Here's how the part is built. I have some questions about the finished solid (model axes, mm). A direction names the side the tool comes from. Coordinates: 2 decimals unless noted, no trailing zeros. Order: outer loops, then holes, each group sorted by start corner. A loop starts at its lowest first (then second) coordinate and runs counter-clockwise, first axis right, second up. Notation, with made-up numbers: (8.25, -39) - (47.25, -39) arc R26 cw to (47.25, -6) - close; hole circle Ø6 at (15.25, 89). An arc over 180 degrees is marked (long way). Answer as CSV lines item,"result". Start each with the question number.
Item 1: Imagine slicing it at C-C on z = -2. List the corners of the cut face in (x, y) for me.
Item 2: Imagine slicing it at A-A on x = 11.5. List the corners of the cut face in (y, z) for me.
Item 3: Imagine slicing it at B-B on y = 2.4. List the corners of the cut face in (x, z) for me.
Item 4: I need wall thicknesses on line 1 (Z direction, x = 11, y = 0.9); line 2 (Z direction, x = 14.5, y = 1.05); line 3 (X direction, y = 2.45, z = -16.5). Which ranges of each line are inside material? Lowest first, please.
Item 5: We'd pull the mould along X, two halves only. Please class faces 5 (the face through (10.762, 1, -62)), 6 (the face through (-18.42, 1.521, -50.347)), 7 (the face through (-19.238, 1, -70)), 8 (the face through (14.566, 1.521, -50.326)): pulls with the +X half, pulls with the -X half, needs draft (parallel to the pull), parting line crosses it, or undercut.
Item 6: I'm going to push flat-ended pins straight in: pin 1 (1.5 mm diameter, centred on y = 1.5, z = -69.5, fed in from +X); pin 2 (1.5 mm diameter, centred on y = 1, z = -9, fed in from -X); pin 3 (3.5 mm diameter, centred on x = -2.74, z = 0.94, fed in from -Y); pin 4 (1.5 mm diameter, centred on x = 12, y = 2, fed in from +Z). Where does each tip first touch, or does it pass through?
Item 7: On a 3-axis mill with a long thin cutter (end or side, diameter ignored), from which of +Z, -Z, +X, -X, +Y, -Y can I reach the whole of each face in a straight line? I mean faces 1 (the face through (14, 1, -56.064)), 2 (the face through (13.762, 1, -70)), 3 (the face through (-19, 1, -44.064)), 4 (the face through (-19, 1, -56.064)). Say none if no direction works.
Autodesk Inventor part; units mm, degrees
ref_plane "YZ Plane" through (0, 0, 0) normal (1, 0, 0) x (0, 1, 0)
ref_plane "XZ Plane" through (0, 0, 0) normal (0, 1, 0) x (-1, 0, 0)
ref_plane "XY Plane" through (0, 0, 0) normal (0, 0, 1) x (1, 0, 0)
sketch "Sketch1" plane through (0, 0, 0) normal (0, 1, 0) x (-1, 0, 0)
  line L0 (16.2379, 4.3509) -> (-10.7621, 4.3509)
  line L1 (-13.7621, -68.0643) -> (-13.7621, -71.0643)
  line L2 (-13.7621, -71.0643) -> (19.2379, -71.0643)
  line L3 (19.2379, -71.0643) -> (19.2379, -68.0643)
  line L4 (22.2379, -56.0643) -> (16.2379, -56.0643)
  line L5 (16.2379, -56.0643) -> (16.2379, -68.0643)
  line L6 (16.2379, -68.0643) -> (19.2379, -68.0643)
  line L7 (-13.7621, -68.0643) -> (-10.7621, -68.0643)
  line L8 (-10.7621, -68.0643) -> (-10.7621, -56.0643)
  line L9 (-10.7621, -56.0643) -> (-16.7621, -56.0643)
  line L10 (22.2379, -56.0643) -> (22.2379, -44.0643)
  line L11 (22.2379, -44.0643) -> (16.2379, -44.0643)
  line L12 (16.2379, -44.0643) -> (16.2379, 4.3509)
  line L13 (-16.7621, -56.0643) -> (-16.7621, -44.0643)
  line L14 (-16.7621, -44.0643) -> (-10.7621, -44.0643)
  line L15 (-10.7621, -44.0643) -> (-10.7621, 4.3509)
  dimension "d8" = 3
  dimension "d9" = 3
  dimension "d11" = 33
  dimension "d12" = 12
  dimension "d13" = 60.4152
  dimension "d14" = 12
  dimension "d24" = 6
  dimension "d25" = 6
extrude "Extrusion1" add sketch "Sketch1" along normal blind 3
sketch "Sketch5" plane through (0, 3, 0) normal (0, 1, 0) x (1, 0, 0)
  circle A0 centre (13.7621, 49.0643) radius 1.496
  circle A1 centre (-19.2379, 49.0643) radius 1.5213
  circle A2 centre (-2.7379, -0.9357) radius 1.5
  line L0 (10.7621, 44.0643) -> (16.7621, 44.0643)
  line L1 (16.7621, 44.0643) -> (16.7621, 56.0643)
  line L2 (-22.2379, 44.0643) -> (-16.2379, 44.0643)
  line L3 (-22.2379, 56.0643) -> (-22.2379, 44.0643)
  line L4 (10.7621, -4.3509) -> (10.7621, 44.0643)
  line L5 (-16.2379, -4.3509) -> (10.7621, -4.3509)
  line L6 (13.7621, 71.0643) -> (-19.2379, 71.0643)
  point P0 (0, 0)
  dimension "d36" = 5
  dimension "d37" = 3
  dimension "d38" = 5
  dimension "d39" = 3
  dimension "d41" = 13.5
  dimension "d42" = 3
  dimension "d46" = 72
extrude "Extrusion2" cut sketch "Sketch5" against normal through all
properties part number "k2_t_l4"
Responses:
1,outline,"(-16.24, 0) - (10.76, 0) - (10.76, 3) - (-16.24, 3) - close"
2,outline,"(0, -71.06) - (3, -71.06) - (3, -68.06) - (0, -68.06) - close; (0, -56.06) - (3, -56.06) - (3, -44.06) - (0, -44.06) - close"
3,outline,"(-22.24, -56.06) - (-16.24, -56.06) - (-16.24, -68.06) - (-19.24, -68.06) - (-19.24, -71.06) - (13.76, -71.06) - (13.76, -68.06) - (10.76, -68.06) - (10.76, -56.06) - (16.76, -56.06) - (16.76, -44.06) - (10.76, -44.06) - (10.76, 4.35) - (-16.24, 4.35) - (-16.24, -44.06) - (-22.24, -44.06) - close; hole circle Ø3.04 at (-19.24, -49.06); hole circle Ø3 at (-2.74, 0.94); hole circle Ø2.99 at (13.76, -49.06)"
4,line 1,"z = -71.06 to -68.06, -56.06 to -44.06"
4,line 2,"z = -56.06 to -50.37, -47.76 to -44.06"
4,line 3,"x = -16.24 to 10.76"
5,face 5,"pulls with the +X half"
5,face 6,"undercut"
5,face 7,"pulls with the -X half"
5,face 8,"undercut"
6,pin 1,"stops at x = 13.76"
6,pin 2,"stops at x = -16.24"
6,pin 3,"stops at y = 0"
6,pin 4,"stops at z = -44.06"
7,face 1,"+X, +Y, -Y"
7,face 2,"-Z, +X, +Y, -Y"
7,face 3,"+Z, -X, +Y, -Y"
7,face 4,"-X, +Y, -Y"
